The listing builds one solid part. Answer for the finished solid, in the listing's coordinates (mm). A direction names the side the tool comes from. Round coordinates to 2 decimals unless told otherwise and drop trailing zeros. Loops run counter-clockwise (first coordinate to the right, second up) from the corner with the lowest first, then second, coordinate; pieces in that order, holes last. Notation, with made-up numbers: (86, 33) -> (99, 33) arc R27 ccw to (99, 67) -> close; hole circle Ø10 at (46.5, 85). An arc over 180 degrees is marked (long way). One line per question, with ' | ' between items.
from build123d import *

# Parameters (mm, degrees)
F0_W      = 300
F0_H      = 500
F1_DEPTH  = 1000
F3_W      = 1000
F3_H      = 500
F3_W_2    = 990
F3_H_2    = 490
F4_DEPTH  = 15
F6_DEPTH  = 25
F7_W      = 120
F7_H      = 100
F8_DEPTH  = 5
F9_W      = 20
F9_H      = 20
F10_DEPTH = 5
F11_W     = 110
F11_H     = 60
F12_DEPTH = 2
F14_R     = 12.5
F15_DEPTH = 6
F16_R     = 2
F17_R     = 3
F18_SIZE  = 1
F19_R     = 1


with BuildPart() as f1:
    # F0 (on Front) → F1 (new body)
    with BuildSketch(Plane.XZ):
        with Locations((150, 250)):
            Rectangle(F0_W, F0_H)
    extrude(amount=F1_DEPTH)

    # F3 (on offset) → F4 (cut)
    with BuildSketch(Plane.YZ.offset(275)):
        with Locations((-500, 250)):
            Rectangle(F3_W, F3_H)
        with Locations((-500, 250)):
            Rectangle(F3_W_2, F3_H_2, mode=Mode.SUBTRACT)
    extrude(amount=-F4_DEPTH, mode=Mode.SUBTRACT)

    # F5 (on face) → F6 (join)
    with BuildSketch(Plane(origin=(0, 0, 0), x_dir=(0, -1, 0), z_dir=(-1, 0, 0))):
        with BuildLine():
            ThreePointArc((250.000000113, 500), (242.9289321482, 482.9289322281), (260, 490))
            ThreePointArc((260, 490), (257.0710678518, 497.0710677719), (250.000000113, 500))
        make_face()
        with BuildLine():
            ThreePointArc((260, 10), (242.9289321881, 17.0710678119), (250, 0))
            ThreePointArc((250, 0), (257.0710678119, 2.9289321881), (260, 10))
        make_face()
        with BuildLine():
            ThreePointArc((760, 10), (742.9289321881, 17.0710678119), (750, 0))
            ThreePointArc((750, 0), (757.0710678119, 2.9289321881), (760, 10))
        make_face()
        with BuildLine():
            ThreePointArc((760, 490), (757.0710678119, 497.0710678119), (750, 500))
            ThreePointArc((750, 500), (742.9289321881, 482.9289321881), (760, 490))
        make_face()
    extrude(amount=F6_DEPTH)

    # F7 (on face) → F8 (join)
    with BuildSketch(Plane.XZ.offset(1000)):
        with Locations((130, 350)):
            Rectangle(F7_W, F7_H)
    extrude(amount=F8_DEPTH)

    # F9 (on face) → F10 (join)
    with BuildSketch(Plane.XZ.offset(1005)):
        with Locations((92.5, 320)):
            Rectangle(F9_W, F9_H)
        with Locations((117.5, 320)):
            Rectangle(F9_W, F9_H)
        with Locations((142.5, 320)):
            Rectangle(F9_W, F9_H)
        with Locations((167.5, 320)):
            Rectangle(F9_W, F9_H)
    extrude(amount=F10_DEPTH)

    # F11 (on face) → F12 (cut)
    with BuildSketch(Plane.XZ.offset(1005)):
        with Locations((130, 365)):
            Rectangle(F11_W, F11_H)
    extrude(amount=-F12_DEPTH, mode=Mode.SUBTRACT)

    # F14 (on face) → F15 (join)
    with BuildSketch(Plane.XZ.offset(1000)):
        with Locations((55, 220)):
            Circle(F14_R)
        with Locations((105, 220)):
            Circle(F14_R)
        with Locations((155, 220)):
            Circle(F14_R)
        with Locations((205, 220)):
            Circle(F14_R)
    extrude(amount=F15_DEPTH)

    # F16
    f16_edges = [f1.edges().sort_by_distance(p)[0] for p in [
        (42.5, -1006, 220),
        (92.5, -1006, 220),
        (142.5, -1006, 220),
        (192.5, -1006, 220),
    ]]
    fillet(f16_edges, radius=F16_R)

    # F17
    f17_edges = [f1.edges().sort_by_distance(p)[0] for p in [
        (70, -1005, 350),
        (130, -1005, 300),
        (190, -1005, 350),
        (130, -1005, 400),
    ]]
    fillet(f17_edges, radius=F17_R)

    # F18
    f18_edges = [f1.edges().sort_by_distance(p)[0] for p in [
        (92.5, -1010, 330),
        (82.5, -1010, 320),
        (92.5, -1010, 310),
        (102.5, -1010, 320),
        (117.5, -1010, 330),
        (107.5, -1010, 320),
        (117.5, -1010, 310),
        (127.5, -1010, 320),
        (142.5, -1010, 330),
        (132.5, -1010, 320),
        (142.5, -1010, 310),
        (152.5, -1010, 320),
        (167.5, -1010, 330),
        (157.5, -1010, 320),
        (167.5, -1010, 310),
        (177.5, -1010, 320),
    ]]
    chamfer(f18_edges, length=F18_SIZE)

    # F19
    f19_edges = [f1.edges().sort_by_distance(p)[0] for p in [
        (130, -1003, 395),
        (75, -1003, 365),
        (130, -1003, 335),
        (185, -1003, 365),
    ]]
    fillet(f19_edges, radius=F19_R)


solid = f1.part
Q1. Find the intervals of material crossed by line 1 (Y direction, x = 14.5, z = 116.5); line 2 (X direction, y = -187, z = 190.5); line 3 (Y direction, x = 153, z = 342), in increasing order. Write a range as from..to.
Numbers:
line 1: -1000..0 | line 2: 0..300 | line 3: -1003..0
Q2. For faces 4 (the face through (287, 0, 254)), 5 (the face through (105, -1006, 220)), 6 (the face through (211.72, -1001.97, 230.54)), determine the directions among +Z, -Z, +X, -X, +Y, -Y from which every point of the face is accessible in a straight line to the end or side of a thin tool.
Numbers:
face 4: +Z, -Z, +X, -X, +Y | face 5: -Z, +X, -X, -Y | face 6: -Y
Q3. For a pull along Z with two mould halves and no side action, classify faces 1 (the face through (287, -493, 500)), 2 (the face through (142, -1010, 320)), 3 (the face through (129, -1003, 365)) as pulls with the +Z half, pulls with the -Z half, needs draft (parallel to the pull), parting line crosses it, or undercut.
Numbers:
face 1: pulls with the +Z half | face 2: needs draft | face 3: undercut
Q4. A cutting plane is placed at B-B on z = 165. Give the vertices of the cut face in (x, y), plus the area to 3 significant figures.
Numbers:
outline: (0, -1000) -> (260, -1000) -> (260, -995) -> (275, -995) -> (275, -1000) -> (300, -1000) -> (300, 0) -> (275, 0) -> (275, -5) -> (260, -5) -> (260, 0) -> (0, 0) -> close | area: 300,000 mm^2
Q5. A cutting plane is placed at A-A on y = -781. Give the vertices of the cut face in (x, z).
Numbers:
outline: (0, 0) -> (260, 0) -> (260, 5) -> (275, 5) -> (275, 0) -> (300, 0) -> (300, 500) -> (275, 500) -> (275, 495) -> (260, 495) -> (260, 500) -> (0, 500) -> close
Q6. Given pin 1 Ø23 at (x, z) = (208.5, 219.5) entering from -Y; pin 2 Ø6 at (x, z) = (51, 333) entering from -Y; pin 3 Ø4 at (x, z) = (209.5, 145.5) entering from +Y; pin 4 Ø2 at (y, z) = (-876.5, 128) entering from -X, each flat-ended and moving along its own axis, determine where each tip first touches the part or whether it passes through.
Numbers:
pin 1: y = -1006 | pin 2: y = -1000 | pin 3: y = 0 | pin 4: x = 0
